from build123d import *

# Parameters (mm, degrees)
SKETCH1_W           = 15
SKETCH1_H           = 20
BOSS_EXTRUDE1_DEPTH = 20
FILLET1_R           = 7.5
CUT_EXTRUDE1_START  = -4.75
SKETCH3_R           = 8.5
CUT_EXTRUDE1_DEPTH  = 10.5
SKETCH4_R           = 2.5
CUT_EXTRUDE2_DEPTH  = 30.261749777
CUT_EXTRUDE3_DEPTH  = 3
SKETCH6_R           = 4
CUT_EXTRUDE4_DEPTH  = 3
SKETCH7_W           = 105
SKETCH7_H           = 80
BOSS_EXTRUDE2_DEPTH = 15
SKETCH9_W           = 101
SKETCH9_H           = 74
CUT_EXTRUDE5_DEPTH  = 10
CUT_EXTRUDE6_DEPTH  = 132.624465811
CUT_EXTRUDE7_START  = -1
CUT_EXTRUDE7_DEPTH  = 2.5
SKETCH13_R          = 1.5
CUT_EXTRUDE8_DEPTH  = 7


with BuildPart() as part:
    # Sketch1 → Boss-Extrude1 (new, symmetric)
    with BuildSketch(Plane.XY):
        Rectangle(SKETCH1_W, SKETCH1_H)
    extrude(amount=BOSS_EXTRUDE1_DEPTH, both=True)

    # Fillet1
    fillet1_edges = [part.edges().sort_by_distance(p)[0] for p in [
        (-7.5, 0, -20),
        (7.5, 0, -20),
    ]]
    fillet(fillet1_edges, radius=FILLET1_R - 0.0001)  # a hair under: the kernel refuses the full size

    # Sketch3 → Cut-Extrude1 (cut)
    with BuildSketch(Plane(origin=(0, 10, 0), x_dir=(1, 0, 0), z_dir=(0, 1, 0)).offset(CUT_EXTRUDE1_START)):
        with Locations((0, 12.5)):
            Circle(SKETCH3_R)
    extrude(amount=-CUT_EXTRUDE1_DEPTH, mode=Mode.SUBTRACT)

    # Sketch4 → Cut-Extrude2 (cut, through all)
    with BuildSketch(Plane(origin=(0, 10, 0), x_dir=(1, 0, 0), z_dir=(0, 1, 0))):
        with Locations(Location((0, 12.5, 0), (0, 0, 270))):
            Circle(SKETCH4_R)
    extrude(amount=-CUT_EXTRUDE2_DEPTH, mode=Mode.SUBTRACT)

    # Sketch5 → Cut-Extrude3 (cut)
    with BuildSketch(Plane(origin=(0, -10, 0), x_dir=(-1, 0, 0), z_dir=(0, -1, 0))):
        Polygon((-2.020725942, 16), (-4.041451884, 12.5), (-2.020725942, 9), (2.020725942, 9), (4.041451884, 12.5), (2.020725942, 16), align=None)
    extrude(amount=-CUT_EXTRUDE3_DEPTH, mode=Mode.SUBTRACT)

    # Sketch6 → Cut-Extrude4 (cut)
    with BuildSketch(Plane(origin=(0, 10, 0), x_dir=(1, 0, 0), z_dir=(0, 1, 0))):
        with Locations(Location((0, 12.5, 0), (0, 0, 270))):
            Circle(SKETCH6_R)
    extrude(amount=-CUT_EXTRUDE4_DEPTH, mode=Mode.SUBTRACT)

    # Sketch7 → Boss-Extrude2 (add)
    with BuildSketch(Plane.ZY.offset(7.5)):
        with Locations((72.5, 0)):
            Rectangle(SKETCH7_W, SKETCH7_H)
    extrude(amount=-BOSS_EXTRUDE2_DEPTH)

    # Sketch9 → Cut-Extrude5 (cut)
    with BuildSketch(Plane(origin=(7.5, 0, 0), x_dir=(0, 0, -1), z_dir=(1, 0, 0))):
        with Locations((-74.5, 0)):
            Rectangle(SKETCH9_W, SKETCH9_H)
    extrude(amount=-CUT_EXTRUDE5_DEPTH, mode=Mode.SUBTRACT)

    # Sketch10 → Cut-Extrude6 (cut, through all)
    with BuildSketch(Plane(origin=(-2.5, 0, 0), x_dir=(0, 0, -1), z_dir=(1, 0, 0))):
        Polygon((-111.773976664, -32), (-74.5, -2.54895671), (-37.226023336, -32), align=None)
        Polygon((-115, -29.45104329), (-77.726023336, 0), (-115, 29.45104329), align=None)
        Polygon((-37.226023336, 32), (-111.773976664, 32), (-74.5, 2.54895671), align=None)
        Polygon((-71.273976664, 0), (-34, 29.45104329), (-34, -29.45104329), align=None)
    extrude(amount=-CUT_EXTRUDE6_DEPTH, mode=Mode.SUBTRACT)

    # Sketch12 → Cut-Extrude7 (cut)
    with BuildSketch(Plane(origin=(0, 10, 0), x_dir=(1, 0, 0), z_dir=(0, 1, 0)).offset(CUT_EXTRUDE7_START)):
        Polygon((-1.58771324, 8.25), (-3.175426481, 5.5), (-1.58771324, 2.75), (1.58771324, 2.75), (7.5, 2.75), (7.5, 8.25), (1.58771324, 8.25), align=None)
    extrude(amount=-CUT_EXTRUDE7_DEPTH, mode=Mode.SUBTRACT)

    # Sketch13 → Cut-Extrude8 (cut)
    with BuildSketch(Plane(origin=(0, 10, 0), x_dir=(1, 0, 0), z_dir=(0, 1, 0))):
        with Locations(Location((0, 5.5, 0), (0, 0, 270))):
            Circle(SKETCH13_R)
    extrude(amount=-CUT_EXTRUDE8_DEPTH, mode=Mode.SUBTRACT)


solid = part.part
Source: CAD feature listing. Evaluate the final solid. Frame: model axes, mm. A direction names the side the tool comes from. Coordinates: 2 decimals unless noted, no trailing zeros. Loops run counter-clockwise (first coordinate to the right, second up) from the corner with the lowest first, then second, coordinate; pieces in that order, holes last. Notation, with made-up numbers: (14.25, 21.5) - (36.25, 21.5) arc R24 ccw to (36.25, 31.5) - close; hole circle Ø11 at (-32, -10.5). An arc over 180 degrees is marked (long way). One line per item, written item: value. Start each with the question number.
1. Section C-C (z = 35.5). Return the cut outline in (x, y), and give its area (3 significant figures).
2. Section B-B (y = -17.5). Return the cut outline in (x, z), and give its area (3 significant figures).
3. Section D-D (y = -34.5). Return the cut outline in (x, z).
4. Section A-A (z = 53). Return the cut outline in (x, y).
5. Ray query, L1, parallel to X at y = -6.2, z = -12.5; L2, parallel to Y at x = -1, z = 113; L3, parallel to Y at x = -5.5, z = 47. Return the intervals inside material, ascending.
6. Contact query for flat-ended pins moving along their axis: P1, Ø1.5, axis at x = -1.5, y = -16.5, coming from the -Z side; P2, Ø6, axis at x = 2.5, z = -4.5, coming from the -Y side; P3, Ø0.8, axis at x = 3, y = 7.5, coming from the +Z side. Output: stop coordinate, or through.
7. Mould query, pull axis X, two halves, no side actions, for faces 1 (the flat face through (-4.96, -17.48, 93.4)), 2 (the flat face through (-2.5, 1, 75)), 3 (the flat face through (-3.045, -8.521, -14.226)). Classes: pulls with the +X half, pulls with the -X half, needs draft (parallel to the pull), parting line crosses it, or undercut.
8. Set-up query: faces 4 (the flat face through (0, -10, 0)), 5 (the flat face through (3, 9, -6)), 6 (the flat face through (2, -5.25, -10)). Return all of +Z, -Z, +X, -X, +Y, -Y with unobstructed straight access to the full face (end or side cutting, diameter ignored); none if empty.
Verdict:
1. outline: (-7.5, -40) - (7.5, -40) - (7.5, -37) - (-2.5, -37) - (-2.5, -28.27) - (-7.5, -28.27) - close; (-7.5, 28.27) - (-2.5, 28.27) - (-2.5, 37) - (7.5, 37) - (7.5, 40) - (-7.5, 40) - close
1. area: 177 mm2
2. outline: (-7.5, 20) - (7.5, 20) - (7.5, 24) - (-2.5, 24) - (-2.5, 34) - (-7.5, 34) - close; (-7.5, 49.13) - (-2.5, 49.13) - (-2.5, 55.58) - (-7.5, 55.58) - close; (-7.5, 93.42) - (-2.5, 93.42) - (-2.5, 99.87) - (-7.5, 99.87) - close; (-7.5, 115) - (-2.5, 115) - (-2.5, 125) - (-7.5, 125) - close
2. area: 225 mm2
3. outline: (-7.5, 20) - (7.5, 20) - (7.5, 24) - (-2.5, 24) - (-2.5, 125) - (-7.5, 125) - close
4. outline: (-7.5, -40) - (7.5, -40) - (7.5, -37) - (-2.5, -37) - (-2.5, -32) - (-7.5, -32) - close; (-7.5, -19.54) - (-2.5, -19.54) - (-2.5, -14.44) - (-7.5, -14.44) - close; (-7.5, 14.44) - (-2.5, 14.44) - (-2.5, 19.54) - (-7.5, 19.54) - close; (-7.5, 32) - (-2.5, 32) - (-2.5, 37) - (7.5, 37) - (7.5, 40) - (-7.5, 40) - close
5. L1: x = -7.5 to -2.5, 2.5 to 7.5
5. L2: y = -40 to -37, 37 to 40
5. L3: y = -40 to -32, -24.28 to -19.18, 19.18 to 24.28, 32 to 40
6. P1: stops at z = 20
6. P2: stops at y = -10
6. P3: stops at z = 24
7. face 1: needs draft
7. face 2: pulls with the +X half
7. face 3: undercut
8. face 4: -Z, +X, -X, -Y
8. face 5: +X
8. face 6: -Z
